Part model, mm, in its own coordinate system. A direction names the side the tool comes from. Coordinates: 2 decimals unless noted, no trailing zeros. Loops run counter-clockwise (first coordinate to the right, second up) from the corner with the lowest first, then second, coordinate; pieces in that order, holes last.
```python
from build123d import *


with BuildPart() as part:
    # Sketch4 → Revolve1 (revolve)
    with BuildSketch(Plane(origin=(0, 0, 0), x_dir=(1, 0, 0), z_dir=(0, 1, 0))):
        with BuildLine():
            Line((-10.933333333, -10.966666667), (-9.933333333, -10.966666667))
            Line((-9.933333333, -10.966666667), (-9.933333333, 4.033333333))
            Line((-9.933333333, 4.033333333), (-8.890939345, 5.63491013))
            Line((-8.890939345, 5.63491013), (-0.702775901, 5.63491013))
            Line((-0.702775901, 5.63491013), (0.339618087, 4.033333333))
            Line((0.339618087, 4.033333333), (4.562176814, -19.592288305))
            Line((4.562176814, -19.592288305), (8.562176814, -19.592288305))
            Line((8.562176814, -19.592288305), (8.562176814, -17.592288305))
            ThreePointArc((8.562176814, -17.592288305), (8.256127983, -15.155893912), (8.330597185, -12.701481994))
            Line((8.330597185, -12.701481994), (4.330597185, -12.701481994))
            Line((4.330597185, -12.701481994), (1.339618087, 4.033333333))
            Line((1.339618087, 4.033333333), (-0.296857623, 6.547681609))
            Line((-0.296857623, 6.547681609), (-9.296857623, 6.547681609))
            Line((-9.296857623, 6.547681609), (-10.933333333, 4.033333333))
            Line((-10.933333333, 4.033333333), (-10.933333333, -10.966666667))
        make_face()
    revolve(axis=Axis((24.066666667, 0, -10.345988756), (0, 0, 1)))


solid = part.part
```
Q1. Saw through at C-C (z = 15). List the corners of the cut face in (x, y), plus the area to 3 significant figures.
Q2. Tool access for faces 1 (the flat face through (19, -25, -5.635)), 2 (the flat face through (9, 6, 12.701)), 3 (the cylindrical face through (26.09, -15.37, 18.58)): list every direction of +Z, -Z, +X, -X, +Y, -Y with a clear straight run to the whole face (end or side of a thin tool).
Q3. Probe line 1 (X direction, y = 15.5, z = -3.5); line 2 (X direction, y = -8, z = 1.25); line 3 (Y direction, x = 26, z = 9.5). List the from-to ranges inside material, lowest first.
Q4. Mould opens along X. For faces 4 (the flat face through (26, 25, -6.548)), 5 (the cylindrical face through (51.84, 21.3, 3.57)), 6 (the cylindrical face through (-8.363, -10.213, 3.362)) say: released by +X, released by -X, zero draft, split by the parting line, or undercut.
Q5. Saw through at D-D (z = 5.75). List the corners of the cut face in (x, y), plus the area to 3 significant figures.
Q6. Drop flat-ended pins along their axis: P1, Ø12, axis at x = 21, z = 16.5, coming from the +Y side; P2, Ø4, axis at x = 25, z = 10.5, coming from the -Y side; P3, Ø1.5, axis at y = -7.5, z = 6, coming from the +X side. Give the stop position or say it passes through.
Q7. Saw through at B-B (z = -1.75). List the corners of the cut face in (x, y).
Checked values:
1. outline: circle Ø40.65 at (24.07, 0); hole circle Ø31.63 at (24.07, 0)
1. area: 512 mm2
2. face 1: +Z
2. face 2: -Z
2. face 3: +Z, -Z
3. line 1: x = -7.31 to -6.19, 6.23 to 7.58, 40.56 to 41.91, 54.33 to 55.45
3. line 2: x = -10.01 to -8.98, 2.73 to 3.81, 44.33 to 45.4, 57.11 to 58.14
3. line 3: y = -34.95 to -33.94, -21.22 to -20.22, 20.22 to 21.22, 33.94 to 34.95
4. face 4: zero draft
4. face 5: split by the parting line
4. face 6: undercut
5. outline: circle Ø70 at (24.07, 0); circle Ø43.96 at (24.07, 0); hole circle Ø68 at (24.07, 0); hole circle Ø41.96 at (24.07, 0)
5. area: 352 mm2
6. P1: stops at y = 34.99
6. P2: stops at y = -35
6. P3: stops at x = 58.41
7. outline: circle Ø70 at (24.07, 0); circle Ø46.64 at (24.07, 0); hole circle Ø68 at (24.07, 0); hole circle Ø44.64 at (24.07, 0)
